Source: CAD feature listing. Evaluate the final solid. Frame: model axes, mm. A direction names the side the tool comes from. Give positions to 0.01 mm unless a question says otherwise; leave off trailing zeros. Loops run counter-clockwise (first coordinate to the right, second up) from the corner with the lowest first, then second, coordinate; pieces in that order, holes last. Notation, with made-up numbers: (72.25, 68.25) - (130.25, 68.25) arc R23 cw to (130.25, 86.25) - close; hole circle Ø7 at (70, 69). An arc over 180 degrees is marked (long way). Put each result on its own line as item: value.
```python
from build123d import *

# Parameters (mm, degrees)
BOSS_EXTRUDE1_DEPTH = 62.5
SKETCH3_R           = 10
CUT_EXTRUDE1_DEPTH  = 125
SKETCH4_W           = 50
SKETCH4_H           = 25
CUT_EXTRUDE2_DEPTH  = 10
SKETCH5_W           = 50
SKETCH5_H           = 25
CUT_EXTRUDE3_DEPTH  = 10


with BuildPart() as part:
    # Sketch2 → Boss-Extrude1 (new body, symmetric)
    with BuildSketch(Plane.XY):
        Polygon((-17.5, 60), (17.5, 60), (30, 10), (80, 10), (80, 0), (22.192235936, 0), (9.692235936, 50), (0, 50), (-9.692235936, 50), (-22.192235936, 0), (-80, 0), (-80, 10), (-30, 10), align=None)
    extrude(amount=BOSS_EXTRUDE1_DEPTH, both=True)

    # Sketch3 → Cut-Extrude1 (cut)
    with BuildSketch(Plane(origin=(0, 10, 0), x_dir=(1, 0, 0), z_dir=(0, 1, 0))):
        with Locations((55, 37.5)):
            Circle(SKETCH3_R)
        with Locations((-55, 37.5)):
            Circle(SKETCH3_R)
        with Locations((-55, -37.5)):
            Circle(SKETCH3_R)
        with Locations((55, -37.5)):
            Circle(SKETCH3_R)
    extrude(amount=-CUT_EXTRUDE1_DEPTH, mode=Mode.SUBTRACT)

    # Sketch4 → Cut-Extrude2 (cut)
    with BuildSketch(Plane(origin=(30.588235294, 7.647058824, 0), x_dir=(0, 0, -1), z_dir=(0.9701425, 0.242535625, 0))):
        with Locations((0, 26.464176571)):
            Rectangle(SKETCH4_W, SKETCH4_H)
    extrude(amount=-CUT_EXTRUDE2_DEPTH, mode=Mode.SUBTRACT)

    # Sketch5 → Cut-Extrude3 (cut)
    with BuildSketch(Plane(origin=(-30.588235294, 7.647058824, 0), x_dir=(0, 0, 1), z_dir=(-0.9701425, 0.242535625, 0))):
        with Locations((0, 26.464176571)):
            Rectangle(SKETCH5_W, SKETCH5_H)
    extrude(amount=-CUT_EXTRUDE3_DEPTH, mode=Mode.SUBTRACT)


solid = part.part
```
1) Mould query, pull axis Y, two halves, no side actions, for faces 1 (the flat face through (-80, 5, 1)), 2 (the flat face through (52, 0, 1)), 3 (the flat face through (-19, 32, -25)). Classes: pulls with the +Y half, pulls with the -Y half, needs draft (parallel to the pull), parting line crosses it, or undercut.
Check result:
face 1: needs draft
face 2: pulls with the -Y half
face 3: undercut
2) Access query for faces 4 (the flat face through (16.355, 44.252, 0.35)), 5 (the flat face through (-22.42, 20, -0.35)), 6 (the flat face through (18.808, 13.539, 0.875)). Directions: +Z, -Z, +X, -X, +Y, -Y. A direction counts if a zero-diameter tool reaches every point of the face in a straight line with its end or side. Return the directions, or none.
Check result:
face 4: +X
face 5: none
face 6: +Z, -Z, -Y
3) Section query C-C, the plane x = 55. Output: boundary loops of the cut face in (y, z), plus the area to 3 significant figures.
Check result:
outline: (0, -62.5) - (10, -62.5) - (10, -47.5) - (0, -47.5) - close; (0, -27.5) - (10, -27.5) - (10, 27.5) - (0, 27.5) - close; (0, 47.5) - (10, 47.5) - (10, 62.5) - (0, 62.5) - close
area: 850 mm²
4) Section query D-D, the plane y = 28.5. Output: boundary loops of the cut face in (x, z) (3 decimals), plus the area to 3 significant figures.
Check result:
outline: (-25.375, -62.5) - (-15.067, -62.5) - (-15.067, -25) - (-25.375, -25) - close; (-25.375, 25) - (-15.067, 25) - (-15.067, 62.5) - (-25.375, 62.5) - close; (15.067, -62.5) - (25.375, -62.5) - (25.375, -25) - (15.067, -25) - close; (15.067, 25) - (25.375, 25) - (25.375, 62.5) - (15.067, 62.5) - close
area: 1,550 mm²
5) Section query B-B, the plane y = 6. Output: boundary loops of the cut face in (x, z), plus the area to 3 significant figures.
Check result:
outline: (-80, -62.5) - (-20.69, -62.5) - (-20.69, 62.5) - (-80, 62.5) - close; (20.69, -62.5) - (80, -62.5) - (80, 62.5) - (20.69, 62.5) - close; hole circle Ø20 at (-55, -37.5); hole circle Ø20 at (-55, 37.5); hole circle Ø20 at (55, -37.5); hole circle Ø20 at (55, 37.5)
area: 13,600 mm²
6) Section query A-A, the plane z = -8. Output: boundary loops of the cut face in (x, y).
Check result:
outline: (-80, 0) - (-22.19, 0) - (-17.5, 18.77) - (-27.2, 21.19) - (-30, 10) - (-80, 10) - close; (-21.14, 45.45) - (-11.44, 43.02) - (-9.69, 50) - (9.69, 50) - (11.44, 43.02) - (21.14, 45.45) - (17.5, 60) - (-17.5, 60) - close; (17.5, 18.77) - (22.19, 0) - (80, 0) - (80, 10) - (30, 10) - (27.2, 21.19) - close
7) Material intervals for line 1 along Z through (x, y) = (-55, 6); line 2 along X through (y, z) = (3, 37.5); line 3 along X through (y, z) = (7, 37), sorted ascending. Write a range as [from, to].
Check result:
line 1: [-62.5, -47.5], [-27.5, 27.5], [47.5, 62.5]
line 2: [-80, -65], [-45, -21.44], [21.44, 45], [65, 80]
line 3: [-80, -64.99], [-45.01, -20.44], [20.44, 45.01], [64.99, 80]
8) Pin query (flat end, axial travel): P1, Ø1, axis at x = 42.5, z = 41.5, coming from the +Y side; P2, Ø12, axis at x = -55, z = -37.5, coming from the -Y side; P3, Ø10, axis at y = 17.5, z = 44, coming from the +X side (3 decimals); P4, Ø6, axis at x = 4, z = -23, coming from the -Y side. Return the tip coordinate at first contact, or that it passes through.
Check result:
P1: y = 10
P2: through
P3: x = 29.375
P4: y = 50
